The model under review builds one solid part; all positions refer to its coordinate system, in mm. A direction names the side the tool comes from. Coordinates: 2 decimals unless noted, no trailing zeros. Loops run counter-clockwise (first coordinate to the right, second up) from the corner with the lowest first, then second, coordinate; pieces in that order, holes last. Notation, with made-up numbers: (7, -7) - (47, -7) arc R18 ccw to (47, 27) - close; hole circle Ø11 at (61, 15). An arc over 180 degrees is marked (long way). One line per item, written item: value. Start each with the question number.
1. To check wall thickness, follow line 1 (X direction, y = 6.25, z = 1.4); line 2 (X direction, y = 3.75, z = 1.7); line 3 (Y direction, x = -12.7, z = 2). State the ranges of each line that lie inside material, in increasing order.
2. For faces 5 (the face through (-64, 0, 0)), 6 (the face through (-48.217, -6.851, 1.565)), list the 3-axis set-ups (+Z, -Z, +X, -X, +Y, -Y) from which the entire face can be reached by the end or side of a thin tool; tool diameter is ignored.
3. We need section D-D, the plane x = -22.5. Give the boundary of the cut face in (y, z) (3 decimals), then the cut area to 3 significant figures.
4. Mouldability with a two-part tool opening along X and no side actions: class faces 1 (the face through (0, 0, 2)), 2 (the face through (-64, 0, 3.175)), 3 (the face through (-78.823, -6.71, 1.565)), 4 (the face through (-31.8, 0, 1.6)) as +X half, -X half, draft (parallel to the pull), parting line (faces both ways), or undercut.
5. We need section B-B, the plane z = 0.5. Count the separate pieces of the cut face and the enclosed holes in it, then the cut area to 3 significant figures.
6. We need section A-A, the plane y = 6.35. Give the boundary of the cut face in (x, z) (3 decimals).
from build123d import *

# Parameters (mm, degrees)
F1_DEPTH = 3.175
F3_D     = 6.7564


# Not quite as in the source:
# - a feature names something its author has since deleted; it is built from what else it names


with BuildPart() as f1:
    # F0 (on Top) → F1 (new body)
    with BuildSketch(Plane.XY):
        with BuildLine():
            Line((0, 0), (0, 12.7))
            Line((0, 12.7), (-127, 12.7))
            Line((-127, 12.7), (-127, 0))
            Line((-127, 0), (-127, -12.7))
            ThreePointArc((-127, -12.7), (-126.2841905951, -12.4607975068), (-125.8560005402, -11.839303972))
            Line((-125.8560005402, -11.839303972), (-122.9379989196, -1.7213920559))
            ThreePointArc((-122.9379989196, -1.7213920559), (-120.65, 0), (-118.3620010804, -1.7213920559))
            Line((-118.3620010804, -1.7213920559), (-115.4439994598, -11.839303972))
            ThreePointArc((-115.4439994598, -11.839303972), (-115.0158094049, -12.4607975068), (-114.3, -12.7))
            ThreePointArc((-114.3, -12.7), (-113.5841905951, -12.4607975068), (-113.1560005402, -11.839303972))
            Line((-113.1560005402, -11.839303972), (-110.2379989196, -1.7213920559))
            ThreePointArc((-110.2379989196, -1.7213920559), (-107.95, 0), (-105.6620010804, -1.7213920559))
            Line((-105.6620010804, -1.7213920559), (-102.7439994598, -11.839303972))
            ThreePointArc((-102.7439994598, -11.839303972), (-102.3158094049, -12.4607975068), (-101.6, -12.7))
            ThreePointArc((-101.6, -12.7), (-100.8841905951, -12.4607975068), (-100.4560005402, -11.839303972))
            Line((-100.4560005402, -11.839303972), (-97.5379989196, -1.7213920559))
            ThreePointArc((-97.5379989196, -1.7213920559), (-95.25, 0), (-92.9620010804, -1.7213920559))
            Line((-92.9620010804, -1.7213920559), (-90.0439994598, -11.839303972))
            ThreePointArc((-90.0439994598, -11.839303972), (-89.6158094049, -12.4607975068), (-88.9, -12.7))
            ThreePointArc((-88.9, -12.7), (-88.1841905951, -12.4607975068), (-87.7560005402, -11.839303972))
            Line((-87.7560005402, -11.839303972), (-84.8379989196, -1.7213920559))
            ThreePointArc((-84.8379989196, -1.7213920559), (-82.55, 0), (-80.2620010804, -1.7213920559))
            Line((-80.2620010804, -1.7213920559), (-77.3439994598, -11.839303972))
            ThreePointArc((-77.3439994598, -11.839303972), (-76.9158094049, -12.4607975068), (-76.2, -12.7))
            ThreePointArc((-76.2, -12.7), (-75.4841905951, -12.4607975068), (-75.0560005402, -11.839303972))
            Line((-75.0560005402, -11.839303972), (-72.1379989196, -1.7213920559))
            ThreePointArc((-72.1379989196, -1.7213920559), (-69.85, 0), (-67.5620010804, -1.7213920559))
            Line((-67.5620010804, -1.7213920559), (-64.6439994598, -11.839303972))
            ThreePointArc((-64.6439994598, -11.839303972), (-64.2158094049, -12.4607975068), (-63.5, -12.7))
            ThreePointArc((-63.5, -12.7), (-62.7841905951, -12.4607975068), (-62.3560005402, -11.839303972))
            Line((-62.3560005402, -11.839303972), (-59.4379989196, -1.7213920559))
            ThreePointArc((-59.4379989196, -1.7213920559), (-57.15, 0), (-54.8620010804, -1.7213920559))
            Line((-54.8620010804, -1.7213920559), (-51.9439994598, -11.839303972))
            ThreePointArc((-51.9439994598, -11.839303972), (-51.5158094049, -12.4607975068), (-50.8, -12.7))
            ThreePointArc((-50.8, -12.7), (-50.0841905951, -12.4607975068), (-49.6560005402, -11.839303972))
            Line((-49.6560005402, -11.839303972), (-46.7379989196, -1.7213920559))
            ThreePointArc((-46.7379989196, -1.7213920559), (-44.45, 0), (-42.1620010804, -1.7213920559))
            Line((-42.1620010804, -1.7213920559), (-39.2439994598, -11.839303972))
            ThreePointArc((-39.2439994598, -11.839303972), (-38.8158094049, -12.4607975068), (-38.1, -12.7))
            ThreePointArc((-38.1, -12.7), (-37.3841905951, -12.4607975068), (-36.9560005402, -11.839303972))
            Line((-36.9560005402, -11.839303972), (-34.0379989196, -1.7213920559))
            ThreePointArc((-34.0379989196, -1.7213920559), (-31.75, 0), (-29.4620010804, -1.7213920559))
            Line((-29.4620010804, -1.7213920559), (-26.5439994598, -11.839303972))
            ThreePointArc((-26.5439994598, -11.839303972), (-26.1158094049, -12.4607975068), (-25.4, -12.7))
            ThreePointArc((-25.4, -12.7), (-24.6841905951, -12.4607975068), (-24.2560005402, -11.839303972))
            Line((-24.2560005402, -11.839303972), (-21.3379989196, -1.7213920559))
            ThreePointArc((-21.3379989196, -1.7213920559), (-19.05, 0), (-16.7620010804, -1.7213920559))
            Line((-16.7620010804, -1.7213920559), (-13.8439994598, -11.839303972))
            ThreePointArc((-13.8439994598, -11.839303972), (-13.4158094049, -12.4607975068), (-12.7, -12.7))
            ThreePointArc((-12.7, -12.7), (-11.9841905951, -12.4607975068), (-11.5560005402, -11.839303972))
            Line((-11.5560005402, -11.839303972), (-8.6379989196, -1.7213920559))
            ThreePointArc((-8.6379989196, -1.7213920559), (-6.35, 0), (-4.0620010804, -1.7213920559))
            Line((-4.0620010804, -1.7213920559), (-1.1439994598, -11.839303972))
            ThreePointArc((-1.1439994598, -11.839303972), (-0.7158094049, -12.4607975068), (0, -12.7))
            Line((0, -12.7), (0, 0))
        make_face()
    extrude(amount=F1_DEPTH)

    # F3 (through all)
    with Locations(Plane.XY.offset(3.175)):
        with Locations((-114.3, 6.35), (-63.5, 6.35), (-12.7, 6.35)):
            Hole(F3_D / 2)


solid = f1.part
Findings below:
1. line 1: -127 to -117.68, -110.92 to -66.88, -60.12 to -16.08, -9.32 to 0
1. line 2: -127 to -116.46, -112.14 to -65.66, -61.34 to -14.86, -10.54 to 0
1. line 3: -12.7 to 2.97, 9.73 to 12.7
2. face 5: -Z, +X, -X, +Y, -Y
2. face 6: +Z, -Z, -Y
3. outline: (-5.751, 0) - (12.7, 0) - (12.7, 3.175) - (-5.751, 3.175) - close
3. area: 58.6 mm2
4. face 1: +X half
4. face 2: draft
4. face 3: undercut
4. face 4: undercut
5. separate pieces: 1
5. enclosed holes: 3
5. area: 2,210 mm2
6. outline: (-127, 0) - (-117.678, 0) - (-117.678, 3.175) - (-127, 3.175) - close; (-110.922, 0) - (-66.878, 0) - (-66.878, 3.175) - (-110.922, 3.175) - close; (-60.122, 0) - (-16.078, 0) - (-16.078, 3.175) - (-60.122, 3.175) - close; (-9.322, 0) - (0, 0) - (0, 3.175) - (-9.322, 3.175) - close
